Geometry check sheet. Reference: the model listing, model coordinates, mm. A direction names the side the tool comes from. Round coordinates to 2 decimals unless told otherwise and drop trailing zeros. Write each loop counter-clockwise with the first axis right and the second up, starting at its lowest first coordinate (ties: lowest second). Pieces come first, ordered by that corner, then holes. Notation, with made-up numbers: (17, 33.5) -> (72, 33.5) arc R18 ccw to (72, 58.5) -> close; hole circle Ø2 at (21, 86). An arc over 180 degrees is marked (long way). One line per question, with ' | ' between items.
Solid Edge part; units mm, degrees
sketch "Sketch1" plane through (0, 0, 0) normal (0, -1, 0) x (1, 0, 0)
  line L0 (0, -30) -> (1.5, -30)
  line L1 (1.5, -30) -> (1.5, -12)
  arc A0 (1.5, -11.99) -> (1.5, -12) centre (1.5038, -11.995) ccw
  line L2 (1.5, -11.99) -> (1.5, 0)
  line L3 (1.5, 0) -> (2.85, 0)
  line L4 (2.85, 0) -> (2.85, 0.165)
  arc A1 (1.27, 1.65) -> (2.85, 0.165) centre (-0.3628, -1.6703) cw
  line L5 (0, 1.65) -> (1.27, 1.65)
  dimension "D1" = 1.5
revolve "RevolvedProtrusion1" add sketch "Sketch1" angle 360 about axis through (0, 0, 5) along (0, 0, -1)
sketch "Sketch2" plane through (0, 0, 0) normal (0, -1, 0) x (1, 0, 0)
  line L0 (0, -0.0566) -> (1.1545, 0.61)
  line L1 (1.1545, 0.61) -> (1.1545, 1.65)
  line L2 (1.1545, 1.65) -> (0, 1.65)
revolve "RevolvedCutout1" cut sketch "Sketch2" angle 360 about axis through (0, 0, 5.3) along (0, 0, -1)
sketch "Sketch3" plane through (0, 0, 0) normal (0, 0, -1) x (0, 1, 0)
  arc A0 (-1, 0.577) -> (-1, -0.577) centre (0, 0) ccw
  line L0 (-1, 0.577) -> (-1, -0.577)
extrude "Protrusion1" add sketch "Sketch3" against normal blind 1.65
pattern_circular "Pattern1" count 6 over 360 about axis through (0, 0, 0) along (0, 0, -1) of "Protrusion1"
fillet "Round_1" radius 0.185 1 edges at (-1.27, 0, 1.65)
sketch "Sketch4" plane through (0, 0, 0) normal (0, -1, 0) x (1, 0, 0)
  line L0 (0, 0.9501) -> (1.2122, 1.65)
  line L1 (1.2122, 1.65) -> (0, 1.65)
revolve "RevolvedCutout2" cut sketch "Sketch4" angle 360 about axis through (0, 0, 5.3) along (0, 0, -1)
sketch "Sketch5" plane through (0, 0, 0) normal (0, -1, 0) x (1, 0, 0)
  line L0 (-1.5, 0) -> (-1.5, -0.1)
  line L1 (-1.6, 0) -> (-1.5, 0)
  arc A0 (-1.6, 0) -> (-1.5, -0.1) centre (-1.6, -0.1) cw
revolve "RevolvedProtrusion2" add sketch "Sketch5" angle 360 about axis through (0, 0, -0.5) along (0, 0, 1)
cosmetic_thread "Thread1"
chamfer "Chamfer1" distance 0.3065 angle 45 1 edges at (-1.5, 0, -30)
properties material "Stahl"
(1) Material ranges on line 1 (Z direction, x = 0.95, y = 0.6); line 2 (Z direction, x = 0.7, y = 1.85); line 3 (X direction, y = 0.9, z = -19.5), recorded low to high.
Resolved:
line 1: z = -30 to 1.6 | line 2: z = 0 to 1.2 | line 3: x = -1.2 to 1.2
(2) Access from +Z, -Z, +X, -X, +Y, -Y to the whole of each face (thin tool, end or side, straight path). Record for faces 4 (the cylindrical face through (-1.5, 0.07, -20.72)), 5 (the flat face through (0, 0, -30)), 6 (the flat face through (0, 1, 1)).
Resolved:
face 4: -Z | face 5: -Z, +X, -X, +Y, -Y | face 6: +Z
(3) Draft check along X on faces 1 (the flat face through (0, 2, 0)), 2 (the flat face through (0.87, -0.49, 1.06)), 3 (the cylindrical face through (-1.5, 0.07, -5.96)). Enter one of: +X half, -X half, draft (parallel to the pull), parting line (faces both ways), or undercut.
Resolved:
face 1: draft | face 2: undercut | face 3: parting line
(4) Sectioned sample at A-A on z = -7. Record the cut outline in (x, y).
Resolved:
outline: circle Ø3 at (0, 0)
(5) Go/stop test with flat-tipped pins: pin 1 (1.5 mm diameter, centred on y = 2, z = -14, fed in from -X); pin 2 (0.5 mm diameter, centred on x = 0, z = 1, fed in from +Y); pin 3 (0.9 mm diameter, centred on x = 0, z = 1.5, fed in from -Y). Record where each tip stops, or that it passes through.
Resolved:
pin 1: stops at x = -0.83 | pin 2: stops at y = 2.44 | pin 3: stops at y = -2.15
